Read the model definition and answer for the solid it produces. Units are mm, in the model's axes. Face numbers are marked on the shaded views. Give positions to 0.01 mm unless a question says otherwise; leave off trailing zeros. Loops run counter-clockwise (first coordinate to the right, second up) from the corner with the lowest first, then second, coordinate; pieces in that order, holes last. Notation, with made-up numbers: (15, -30.5) - (45, -30.5) arc R21 ccw to (45, -18.5) - close; hole circle Ø5 at (81, 75). An arc over 180 degrees is marked (long way). Write each question's results on one line, items separated by ' | '. Start each with the question number.
Q1. Given pin 1 (1.4 mm diameter, centred on y = 1, z = -25.5, fed in from -X); pin 2 (1.9 mm diameter, centred on x = -24, z = -16, fed in from +Y); pin 3 (0.5 mm diameter, centred on y = 1, z = -25, fed in from +X), each flat-ended and moving along its own axis, determine where each tip first touches the part or whether it passes through.
Q2. The part is cut by section C-C, the plane z = -4.5. Write down the section's boundary in (x, y), plus the area to 3 significant figures.
Q3. Determine the mould class of the marked faces 1, 2, 3 and 4 for opening direction X: +X half, -X half, draft (parallel to the pull), parting line (faces both ways), or undercut.
Q4. The part is cut by section D-D, the plane y = 9.7. Write down the section's boundary in (x, z).
Q5. The part is cut by section B-B, the plane z = 7. Write down the section's boundary in (x, y), plus the area to 3 significant figures.
Q6. Find the intervals of material crossed by line 1 (Z direction, x = -6, y = 1.25); line 2 (X direction, y = 12.5, z = -4); line 3 (Y direction, x = 2.25, z = 3.5), in increasing order. Write a range as from..to.
Q7. The part is cut by section A-A, the plane x = -6. Write down the section's boundary in (y, z), plus the area to 3 significant figures.
Autodesk Inventor part; units mm, degrees
ref_plane "YZ Plane" through (0, 0, 0) normal (1, 0, 0) x (0, 1, 0)
ref_plane "XZ Plane" through (0, 0, 0) normal (0, 1, 0) x (-1, 0, 0)
ref_plane "XY Plane" through (0, 0, 0) normal (0, 0, 1) x (1, 0, 0)
sketch "Sketch1" plane through (0, 0, 0) normal (0, 1, 0) x (-1, 0, 0)
  line L0 (0, 0) -> (20, 0)
  line L1 (20, 0) -> (20, -40)
  line L2 (20, -40) -> (0, -40)
  line L3 (0, -40) -> (0, 0)
  line L4 (25, 30) -> (-5, 30)
  line L5 (-5, 30) -> (-5, -50)
  line L6 (-5, -50) -> (25, -50)
  line L7 (25, -50) -> (25, 30)
  dimension "d0" = 20
  dimension "d1" = 40
  dimension "d2" = 30
  dimension "d3" = 30
  dimension "d4" = 10
  dimension "d5" = 5
extrude "Extrusion1" add sketch "Sketch1" along normal blind 1.7
sketch "Sketch2" plane through (5, 0, 30) normal (1, 0, 0) x (0, 0, -1)
  line L0 (0, 0) -> (0, 1.7)
  line L1 (0, 1.7) -> (0, 13.7)
  line L2 (0, 13.7) -> (22.5503, 35.1708)
  line L3 (22.5503, 35.1708) -> (56.8462, 35.7913)
  line L4 (56.8462, 35.7913) -> (80, 13.7)
  line L5 (80, 0) -> (80, 1.7)
  line L6 (80, 13.7) -> (80, 1.7)
  line L7 (0, 1.7) -> (80, 1.7)
  circle A0 centre (70.3665, 9.7) radius 1.5
  circle A1 centre (70.3665, 9.7) radius 28
  line L8 (24.8863, 30.7) -> (59.3173, 30.7)
  circle A2 centre (51.8462, 30.7) radius 1.5
  point P0 (30, 0)
  dimension "d11" = 56
  dimension "d8" = 0
  dimension "d9" = 3
  dimension "d10" = 8
  dimension "d12" = 29
  dimension "d13" = 3
  dimension "d14" = 5
  dimension "d15" = 5
  dimension "d16" = 12
  dimension "d19" = 12
extrude "Extrusion2" add sketch "Sketch2" against normal blind 1.7 contours L1 L2 L3 L4 A1 A2 L7 | A1 A2 L4 L6 L7
sketch "Sketch3" plane through (-25, 0, -50) normal (-1, 0, 0) x (0, 0, 1)
  line L0 (0, 0) -> (0, 13.7)
  line L1 (23.1538, 35.7913) -> (0, 13.7)
  line L2 (0, 1.667) -> (0, 13.7)
  line L3 (0, 13.7) -> (80, 13.7)
  line L4 (80, 1.7) -> (0, 1.7)
  line L5 (80, 0) -> (80, 1.7)
  line L6 (0, 1.7) -> (80, 1.7)
  line L7 (80, 1.7) -> (80, 13.7)
  circle A0 centre (9.6335, 9.7) radius 1.5
  circle A1 centre (9.6335, 9.7) radius 1.5
  point P0 (50, 0)
  dimension "d20" = 80
  dimension "d21" = 3
extrude "Extrusion3" add sketch "Sketch3" against normal blind 1.7
fillet "Fillet1" radius 2 2 edges at (-25, 0, -10) (5, 0, -10)
fillet "Fillet2" radius 6 6 edges at (4.15, 13.7, 30) (4.15, 35.1708, 7.4497) (4.15, 35.7913, -26.8462) (4.15, 13.7, -50) (-24.15, 13.7, -50) (-24.15, 13.7, 30)
sketch "Sketch4" plane through (0, 1.7, 0) normal (0, 1, 0) x (1, 0, 0)
  line L0 (-6, 47) -> (-14, 47)
  line L1 (-14, 47) -> (-14, -7)
  line L2 (-14, -7) -> (-6, -7)
  line L3 (-6, -7) -> (-6, 47)
  line L4 (-20, 0) -> (-20, 40)
  line L5 (-20, 40) -> (0, 40)
  circle A0 centre (-6, 47) radius 1.5
  circle A1 centre (-14, 47) radius 1.5
  circle A2 centre (-6, -7) radius 1.5
  circle A3 centre (-14, -7) radius 1.5
  point P0 (0, 0)
  point P1 (-10, 40)
  dimension "d26" = 8
  dimension "d27" = 54
  dimension "d28" = 6
  dimension "d29" = 7
  dimension "d30" = 3
  dimension "d31" = 3
  dimension "d32" = 3
  dimension "d33" = 3
extrude "Extrusion4" cut sketch "Sketch4" against normal through all contours A1 L1 L0 | L0 L1 A1 | A0 L3 L0 | L0 L3 A0 | A3 L2 L1 | L1 L2 A3 | A2 L2 L3 | L3 L2 A2
properties part number "gripper servo mount"
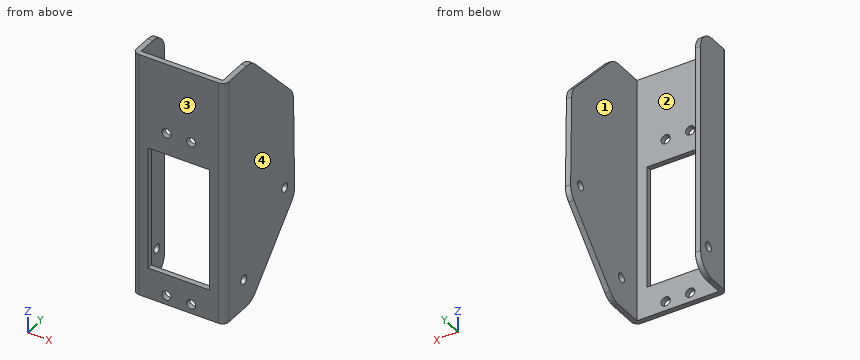
Check sheet entries:
1) pin 1: stops at x = -24.98 | pin 2: stops at y = 13.7 | pin 3: stops at x = 4.85
2) outline: (-25, 2) arc R2 ccw to (-23, 0) - (-20, 0) - (-20, 1.7) - (-23.3, 1.7) - (-23.3, 13.7) - (-25, 13.7) - close; (0, 0) - (3, 0) arc R2 ccw to (5, 2) - (5, 35.39) - (3.3, 35.39) - (3.3, 1.7) - (0, 1.7) - close | area: 93.0 mm^2
3) face 1: undercut | face 2: undercut | face 3: draft | face 4: +X half
4) outline: (-25, -49.66) - (-23.3, -49.66) - (-23.3, -41.87) - (-25, -41.87) - close; (-25, -38.87) - (-23.3, -38.87) - (-23.3, 29.66) - (-25, 29.66) - close; (3.3, -50) - (5, -50) - (5, -41.87) - (3.3, -41.87) - close; (3.3, -38.87) - (5, -38.87) - (5, 30) - (3.3, 30) - close
5) outline: (-25, 2) arc R2 ccw to (-23, 0) - (-15.5, 0) - (-15.5, 1.7) - (-23.3, 1.7) - (-23.3, 13.7) - (-25, 13.7) - close; (-12.5, 0) - (-7.5, 0) - (-7.5, 1.7) - (-12.5, 1.7) - close; (-4.5, 0) - (3, 0) arc R2 ccw to (5, 2) - (5, 34.87) - (3.3, 34.87) - (3.3, 1.7) - (-4.5, 1.7) - close | area: 116 mm^2
6) line 1: z = -50..-48.5, -45.5..-40, 0..5.5, 8.5..30 | line 2: x = -25..-23.3, 3.3..5 | line 3: y = 0..1.7
7) outline: (0, -50) - (1.7, -50) - (1.7, -48.5) - (0, -48.5) - close; (0, -45.5) - (1.7, -45.5) - (1.7, -40) - (0, -40) - close; (0, 0) - (1.7, 0) - (1.7, 5.5) - (0, 5.5) - close; (0, 8.5) - (1.7, 8.5) - (1.7, 30) - (0, 30) - close | area: 57.8 mm^2
